Check sheet for the drawn part. Datum: minimum x, y, z corner. Units: mm. A direction names the side the tool comes from. Give positions to 0.01 mm unless a question says otherwise; leave off trailing zeros. Loops run counter-clockwise (first coordinate to the right, second up) from the corner with the lowest first, then second, coordinate; pieces in that order, holes last. Notation, with made-up numbers: (62.5, 6.25) - (67.5, 6.25) arc R17 cw to (67.5, 22.25) - close; hole circle Ø2 at (15.5, 1). An arc over 180 degrees is marked (long way). One line per item, written item: value. Start each with the question number.
1. Sectioned sample at A-A (y = 54). Record the cut outline in (x, z).
2. Sectioned sample at B-B (x = 65.5). Record the cut outline in (y, z) (3 decimals).
3. Scan lines: L1, parallel to X at y = 28.5, z = 25; L2, parallel to Z at x = 249.5, y = 9; L3, parallel to Y at x = 41.5, z = 17. Record each from-to range of solid material in increasing order. Write a range as [from, to].
4. Mould release check, pull along Y, two halves, no side actions. Record for the marked faces 1, 2 and 3: pulls with the +Y half, pulls with the -Y half, needs draft (parallel to the pull), parting line crosses it, or undercut.
5. Gauge pin test, flat ends, axial feed: pin 1 (24 mm diameter, centred on y = 8, z = 107, fed in from -X); pin 2 (12 mm diameter, centred on x = 19.5, y = 51.5, fed in from -Z); pin 3 (24.5 mm diameter, centred on x = 52.5, z = 71, fed in from +Y); pin 4 (3 mm diameter, centred on x = 36, y = 60, fed in from +Z). Record the tip position at first contact, or that the pin passes through.
6. Access from +Z, -Z, +X, -X, +Y, -Y to the whole of each face (thin tool, end or side, straight path). Record for the marked faces 4, 5, 6, 7 and 8.
7. Sectioned sample at D-D (z = 34.5). Record the cut outline in (x, y).
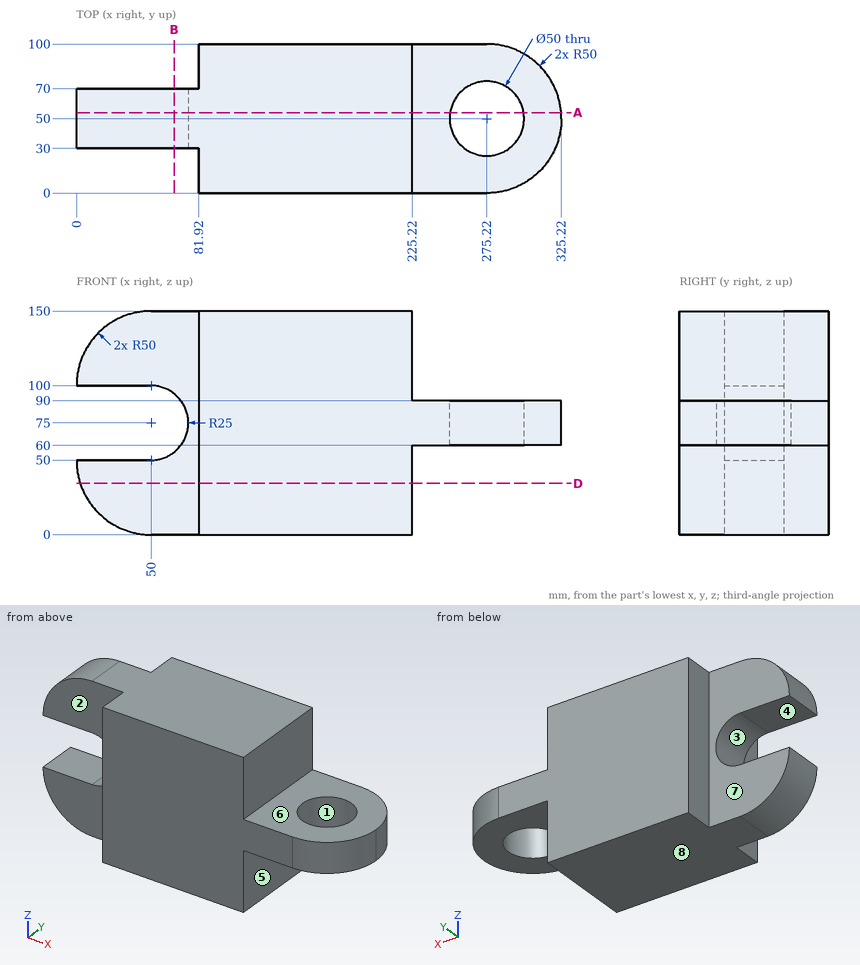
Results are:
1. outline: (0, 50) arc R50 ccw to (50, 0) - (225.22, 0) - (225.22, 60) - (250.54, 60) - (250.54, 90) - (225.22, 90) - (225.22, 150) - (50, 150) arc R50 ccw to (0, 100) - (50, 100) arc R25 cw to (50, 50) - close; (299.9, 60) - (325.06, 60) - (325.06, 90) - (299.9, 90) - close
2. outline: (30, 0) - (70, 0) - (70, 55.385) - (30, 55.385) - close; (30, 94.615) - (70, 94.615) - (70, 150) - (30, 150) - close
3. L1: x = [81.92, 225.22]
3. L2: z = [60, 90]
3. L3: y = [30, 70]
4. face 1: undercut
4. face 2: pulls with the -Y half
4. face 3: needs draft
5. pin 1: stops at x = 81.92
5. pin 2: stops at z = 6.41
5. pin 3: passes through
5. pin 4: stops at z = 148.41
6. face 4: -X, +Y, -Y
6. face 5: -Z, +X, +Y, -Y
6. face 6: +Z, +X, +Y, -Y
6. face 7: +Z, -Z, -X, +Y
6. face 8: -Z, +X, -X, +Y, -Y
7. outline: (2.46, 30) - (81.92, 30) - (81.92, 0) - (225.22, 0) - (225.22, 100) - (81.92, 100) - (81.92, 70) - (2.46, 70) - close
